from build123d import *

# Parameters (mm, degrees)
SKETCH1_R           = 10
BOSS_EXTRUDE1_DEPTH = 12
CUT_EXTRUDE1_DEPTH  = 59.523499554
CUT_EXTRUDE2_START  = 8
CUT_EXTRUDE2_DEPTH  = 4
CUT_EXTRUDE3_DEPTH  = 4
BOSS_EXTRUDE2_START = 6
SKETCH4_R           = 13.5
SKETCH4_R_2         = 12
BOSS_EXTRUDE2_DEPTH = 4.25
SKETCH6_R           = 12
SKETCH6_R_2         = 10
CUT_EXTRUDE4_DEPTH  = 3
CUT_EXTRUDE5_START  = 9
SKETCH6_2_R         = 12
SKETCH6_2_R_2       = 10
CUT_EXTRUDE5_DEPTH  = 3
SKETCH7_R           = 2.5
CUT_EXTRUDE6_DEPTH  = 5
SKETCH8_W           = 10
SKETCH8_H           = 7
CUT_EXTRUDE7_DEPTH  = 2.5
SKETCH9_W           = 24
SKETCH9_H           = 4
CUT_EXTRUDE8_DEPTH  = 1
FILLET1_R           = 1
FILLET2_R           = 2
FILLET3_R           = 1


with BuildPart() as part:
    # Sketch1 → Boss-Extrude1 (new body)
    with BuildSketch(Plane.XY):
        with BuildLine():
            Line((27.5, -16), (-27.5, -16))
            Line((-27.5, -16), (-27.5, -11))
            Line((-27.5, -11), (-13.5, -11))
            Line((-13.5, -11), (-13.5, 0))
            ThreePointArc((-13.5, 0), (0, 13.5), (13.5, 0))
            Line((13.5, 0), (13.5, -11))
            Line((13.5, -11), (27.5, -11))
            Line((27.5, -11), (27.5, -16))
        make_face()
        Circle(SKETCH1_R, mode=Mode.SUBTRACT)
    extrude(amount=BOSS_EXTRUDE1_DEPTH)

    # Sketch2 → Cut-Extrude1 (cut, through all)
    with BuildSketch(Plane.ZY.offset(27.5)):
        Polygon((10.25, 0), (12, -11), (12, 13.5), (10.25, 13.5), align=None)
        Polygon((0, -11), (1.75, 0), (1.75, 13.5), (0, 13.5), align=None)
    extrude(amount=-CUT_EXTRUDE1_DEPTH, mode=Mode.SUBTRACT)

    # Sketch3 → Cut-Extrude2 (cut)
    with BuildSketch(Plane.XY.offset(CUT_EXTRUDE2_START)):
        with BuildLine():
            ThreePointArc((12, 0), (0, -12), (-12, 0))
            Line((-12, 0), (-12, -16))
            Line((-12, -16), (12, -16))
            Line((12, -16), (12, 0))
        make_face()
    extrude(amount=CUT_EXTRUDE2_DEPTH, mode=Mode.SUBTRACT)

    # Sketch3<3> → Cut-Extrude3 (cut)
    with BuildSketch(Plane.XY):
        with BuildLine():
            ThreePointArc((12, 0), (0, -12), (-12, 0))
            Line((-12, 0), (-12, -16))
            Line((-12, -16), (12, -16))
            Line((12, -16), (12, 0))
        make_face()
    extrude(amount=CUT_EXTRUDE3_DEPTH, mode=Mode.SUBTRACT)

    # Sketch4 → Boss-Extrude2 (add, symmetric)
    with BuildSketch(Plane.XY.offset(BOSS_EXTRUDE2_START)):
        Circle(SKETCH4_R)
        Circle(SKETCH4_R_2, mode=Mode.SUBTRACT)
    extrude(amount=BOSS_EXTRUDE2_DEPTH, both=True)

    # Sketch6 → Cut-Extrude4 (cut)
    with BuildSketch(Plane.XY):
        Circle(SKETCH6_R)
        Circle(SKETCH6_R_2, mode=Mode.SUBTRACT)
    extrude(amount=CUT_EXTRUDE4_DEPTH, mode=Mode.SUBTRACT)

    # Sketch6<2> → Cut-Extrude5 (cut)
    with BuildSketch(Plane.XY.offset(CUT_EXTRUDE5_START)):
        Circle(SKETCH6_2_R)
        Circle(SKETCH6_2_R_2, mode=Mode.SUBTRACT)
    extrude(amount=CUT_EXTRUDE5_DEPTH, mode=Mode.SUBTRACT)

    # Sketch7 → Cut-Extrude6 (cut)
    with BuildSketch(Plane.XZ.offset(16)):
        with Locations((-21, 6)):
            Circle(SKETCH7_R)
        with Locations((21, 6)):
            Circle(SKETCH7_R)
    extrude(amount=-CUT_EXTRUDE6_DEPTH, mode=Mode.SUBTRACT)

    # Sketch8 → Cut-Extrude7 (cut)
    with BuildSketch(Plane.XZ.offset(16)):
        with Locations((20, 6)):
            Rectangle(SKETCH8_W, SKETCH8_H)
        with Locations((-20, 6)):
            Rectangle(SKETCH8_W, SKETCH8_H)
    extrude(amount=-CUT_EXTRUDE7_DEPTH, mode=Mode.SUBTRACT)

    # Sketch9 → Cut-Extrude8 (cut)
    with BuildSketch(Plane.XZ.offset(16)):
        with Locations((0, 6)):
            Rectangle(SKETCH9_W, SKETCH9_H)
    extrude(amount=-CUT_EXTRUDE8_DEPTH, mode=Mode.SUBTRACT)

    # Fillet1
    fillet1_edges = [part.edges().sort_by_distance(p)[0] for p in [
        (13.5, -11, 6),
        (-13.5, -11, 6),
        (12, -15, 6),
        (-12, -15, 6),
    ]]
    fillet(fillet1_edges, radius=FILLET1_R - 0.0001)  # a hair under: the kernel refuses the full size

    # Fillet2
    fillet2_edges = [part.edges().sort_by_distance(p)[0] for p in [
        (-27.5, -13.5, 0),
        (-27.5, -13.5, 12),
        (27.5, -13.5, 12),
        (27.5, -13.5, 0),
    ]]
    fillet(fillet2_edges, radius=FILLET2_R)

    # Fillet3
    fillet3_edges = [part.edges().sort_by_distance(p)[0] for p in [
        (-25, -14.75, 9.5),
        (-15, -14.75, 9.5),
        (-15, -14.75, 2.5),
        (-25, -14.75, 2.5),
        (25, -14.75, 9.5),
        (25, -14.75, 2.5),
        (15, -14.75, 2.5),
        (15, -14.75, 9.5),
    ]]
    fillet(fillet3_edges, radius=FILLET3_R)


solid = part.part
Work out the finished part from the listing and answer in its coordinate system (mm). A direction names the side the tool comes from. Coordinates: 2 decimals unless noted, no trailing zeros. Write each loop counter-clockwise with the first axis right and the second up, starting at its lowest first coordinate (ties: lowest second). Pieces come first, ordered by that corner, then holes. Notation, with made-up numbers: (19, 39.5) - (35, 39.5) arc R15 ccw to (35, 50.5) - close; hole circle Ø2 at (21, -37.5). An arc over 180 degrees is marked (long way). One line per question, with ' | ' between items.
1) Find section A-A, the plane x = 0. Determine the outline of the cut face in (y, z).
Checks:
outline: (-15, 4) - (-13.5, 4) - (-13.5, 1.75) - (-12, 1.75) - (-12, 3) - (-10, 3) - (-10, 9) - (-12, 9) - (-12, 10.25) - (-13.5, 10.25) - (-13.5, 8) - (-15, 8) - close; (10, 3) - (12, 3) - (12, 1.75) - (13.5, 1.75) - (13.5, 10.25) - (12, 10.25) - (12, 9) - (10, 9) - close
2) For faces 5 (the face through (-5, 9, 9)), 6 (the face through (-0.1, 12.2, 1.75)), 7 (the face through (-15.301, -14.732, 2.785)), 8 (the face through (11.715, -15.301, 6.028)), determine the directions among +Z, -Z, +X, -X, +Y, -Y from which every point of the face is accessible in a straight line to the end or side of a thin tool.
Checks:
face 5: +Z | face 6: -Z, +X, -X, +Y | face 7: -Y | face 8: +Z, -Z, -Y
3) Find section D-D, the plane x = 21. Determine the outline of the cut face in (y, z), and give its area (3 significant figures).
Checks:
outline: (-16, 0) - (-11, 0) - (-11, 3.5) - (-13.5, 3.5) - (-13.5, 2.5) - (-16, 2.5) - close; (-16, 9.5) - (-13.5, 9.5) - (-13.5, 8.5) - (-11, 8.5) - (-11, 12) - (-16, 12) - close | area: 30.0 mm2
4) The mould has two halves that part along Z. Classify faces 1 (the face through (12.677, -5.423, 11.113)), 2 (the face through (-0.297, 13.497, 5.94)), 3 (the face through (26.93, -13.54, 0.6)), 4 (the face through (-20, -15, 9.5)): +Z half, -Z half, draft (parallel to the pull), parting line (faces both ways), or undercut.
Checks:
face 1: +Z half | face 2: draft | face 3: -Z half | face 4: undercut
5) Consider probe 1 along Y at (x, z) = (0, 4.8); probe 2 along Y at (x, z) = (0, 2.6); probe 3 along Y at (x, z) = (-19, 1). Determine where each line is inside the solid, lowest interval first. Write a range as [from, to].
Checks:
probe 1: [-15, -10], [10, 13.5] | probe 2: [-13.5, -12], [12, 13.5] | probe 3: [-16, -11]
6) Find section C-C, the plane z = 1. Determine the outline of the cut face in (x, y).
Checks:
outline: (-27.23, -16) - (-12, -16) - (-12, -4.71) - (-13.5, -4.71) - (-13.5, -10) arc R1 cw to (-14.5, -11) - (-27.23, -11) - close; (12, -16) - (27.23, -16) - (27.23, -11) - (14.5, -11) arc R1 cw to (13.5, -10) - (13.5, -4.71) - (12, -4.71) - close
7) Flat-ended cylindrical pins translate along their axes: P1, Ø5, axis at x = 3.5, y = 10.5, coming from the -Z side; P2, Ø3.5, axis at x = 18.5, z = 4.5, coming from the -Y side; P3, Ø6, axis at y = 7, z = 9.5, coming from the -X side. Find the tip coordinate at first contact, or state that the pin passes through.
Checks:
P1: z = 1.75 | P2: y = -13.5 | P3: x = -12.89
